```python
from build123d import *

# Parameters (mm, degrees)
SKETCH1_W           = 17
SKETCH1_H           = 30
SKETCH1_R           = 2.5
SKETCH1_W_2         = 40
SKETCH1_R_2         = 2.35
BOSS_EXTRUDE1_DEPTH = 3


with BuildPart() as part:
    # Sketch1 → Boss-Extrude1 (new body)
    # profile 1 of 3: a face of its own
    with BuildSketch(Plane(origin=(0, 0, 0), x_dir=(0, 0, -1), z_dir=(1, 0, 0))):
        with Locations((21.933683822, -2.188772059)):
            Rectangle(SKETCH1_W, SKETCH1_H)
        with Locations((20.433683822, 6.811227941)):
            Circle(SKETCH1_R, mode=Mode.SUBTRACT)
    # profile 2 of 3: a face of its own
    with BuildSketch(Plane(origin=(0, 0, 0), x_dir=(0, 0, -1), z_dir=(1, 0, 0))):
        with Locations((-6.566316178, -2.188772059)):
            Rectangle(SKETCH1_W_2, SKETCH1_H)
        with Locations((-18.566316178, 6.811227941)):
            Circle(SKETCH1_R_2, mode=Mode.SUBTRACT)
        with Locations((5.433683822, 6.811227941)):
            Circle(SKETCH1_R_2, mode=Mode.SUBTRACT)
        with Locations((5.433683822, -11.188772059)):
            Circle(SKETCH1_R_2, mode=Mode.SUBTRACT)
        with Locations((-18.566316178, -11.188772059)):
            Circle(SKETCH1_R_2, mode=Mode.SUBTRACT)
    # profile 3 of 3: a face of its own
    with BuildSketch(Plane(origin=(0, 0, 0), x_dir=(0, 0, -1), z_dir=(1, 0, 0))):
        with Locations((-35.066316178, -2.188772059)):
            Rectangle(SKETCH1_W, SKETCH1_H)
        with Locations((-33.566316178, 6.811227941)):
            Circle(SKETCH1_R, mode=Mode.SUBTRACT)
    extrude(amount=BOSS_EXTRUDE1_DEPTH)


solid = part.part
```
Source: CAD feature listing. Evaluate the final solid. Frame: model axes, mm. Round coordinates to 2 decimals unless told otherwise and drop trailing zeros. Write each loop counter-clockwise with the first axis right and the second up, starting at its lowest first coordinate (ties: lowest second). Pieces come first, ordered by that corner, then holes. Notation, with made-up numbers: M 74.5,81 L 107.5,81 A7 cw 107.5,94 Z; hole C 27.5,-33.5 d7. An arc over 180 degrees is marked long. Use CSV: the item, a comma, the result in double quotes. Start each with the question number.
Q1. Pull-direction query (Z, two-part tool) for faces 1 (the face through (1, -2, 43.566)), 2 (the face through (1, 12.811, 7)), 3 (the face through (1.48, 8.79, -6.7)); classes: +Z half, -Z half, draft (parallel to the pull), parting line (faces both ways), or undercut.
Q2. Cut plane C-C on z = -6. Output: boundary loops of the cut face in (x, y), plus the area to 3 significant figures.
Q3. Line query: line 1 (Z direction, x = 1.85, y = 7); line 2 (Y direction, x = 2.7, z = 18.5); line 3 (Y direction, x = 0.9, z = -7). Output: solid intervals per line, ascending. Write a range as from..to.
Q4. Cut plane A-A on z = 32.5. Output: boundary loops of the cut face in (x, y).
Q5. Cut plane D-D on x = 1.8. Output: boundary loops of the cut face in (y, z).
Q6. Cut plane B-B on y = 5.5. Output: boundary loops of the cut face in (x, z), plus the area to 3 significant figures.
Results found:
1,face 1,"+Z half"
1,face 2,"draft"
1,face 3,"undercut"
2,outline,"M 0,-17.19 L 3,-17.19 L 3,-13.47 L 0,-13.47 Z; M 0,-8.91 L 3,-8.91 L 3,4.53 L 0,4.53 Z; M 0,9.09 L 3,9.09 L 3,12.81 L 0,12.81 Z"
2,area,"62.6 mm^2"
3,line 1,"-30.43..-22.93, -17.94..-7.78, -3.09..16.22, 20.91..31.07, 36.06..43.57"
3,line 2,"-17.19..-13.54, -8.84..4.46, 9.16..12.81"
3,line 3,"-17.19..-12.94, -9.44..5.06, 8.56..12.81"
4,outline,"M 0,-17.19 L 3,-17.19 L 3,4.55 L 0,4.55 Z; M 0,9.07 L 3,9.07 L 3,12.81 L 0,12.81 Z"
5,outline,"M -17.19,-30.43 L 12.81,-30.43 L 12.81,43.57 L -17.19,43.57 Z; hole C -11.19,-5.43 d4.7; hole C -11.19,18.57 d4.7; hole C 6.81,-20.43 d5; hole C 6.81,33.57 d5; hole C 6.81,-5.43 d4.7; hole C 6.81,18.57 d4.7"
6,outline,"M 0,-30.43 L 3,-30.43 L 3,-22.56 L 0,-22.56 Z; M 0,-18.31 L 3,-18.31 L 3,-7.38 L 0,-7.38 Z; M 0,-3.48 L 3,-3.48 L 3,16.62 L 0,16.62 Z; M 0,20.52 L 3,20.52 L 3,31.44 L 0,31.44 Z; M 0,35.69 L 3,35.69 L 3,43.57 L 0,43.57 Z"
6,area,"173 mm^2"
